Read the model definition and answer for the solid it produces. Units are mm, in the model's axes. A direction names the side the tool comes from. Give positions to 0.01 mm unless a question says otherwise; leave off trailing zeros. Loops run counter-clockwise (first coordinate to the right, second up) from the corner with the lowest first, then second, coordinate; pieces in that order, holes last. Notation, with made-up numbers: (84.5, -22) - (111.5, -22) arc R24 ccw to (111.5, 11) - close; hole circle Ø5 at (-3.75, -35). An arc over 180 degrees is marked (long way). Write item = value, one per line.
```python
from build123d import *

# Parameters (mm, degrees)
SKETCH1_W           = 27.4
SKETCH1_H           = 15.5
BOSS_EXTRUDE1_DEPTH = 9.6
FILLET1_R           = 2
SKETCH2_W           = 13
SKETCH2_H           = 4.45
BOSS_EXTRUDE2_DEPTH = 8
SKETCH3_W           = 0.5
SKETCH3_H           = 4.45
BOSS_EXTRUDE3_DEPTH = 35
CHAMFER1_SIZE       = 5
CHAMFER1_SIZE2      = 10.722534603


with BuildPart() as part:
    # Sketch1 → Boss-Extrude1 (new body)
    with BuildSketch(Plane(origin=(0, 0, 0), x_dir=(1, 0, 0), z_dir=(0, 1, 0))):
        with Locations((13.7, 7.75)):
            Rectangle(SKETCH1_W, SKETCH1_H)
    extrude(amount=BOSS_EXTRUDE1_DEPTH)

    # Fillet1
    fillet1_edges = [part.edges().sort_by_distance(p)[0] for p in [
        (0, 4.8, -15.5),
        (27.4, 4.8, -15.5),
        (27.4, 4.8, 0),
        (0, 4.8, 0),
    ]]
    fillet(fillet1_edges, radius=FILLET1_R)

    # Sketch2 → Boss-Extrude2 (add)
    with BuildSketch(Plane(origin=(0, 0, -15.5), x_dir=(-1, 0, 0), z_dir=(0, 0, -1))):
        with Locations((-10.5, 4.875)):
            Rectangle(SKETCH2_W, SKETCH2_H)
    extrude(amount=BOSS_EXTRUDE2_DEPTH)

    # Sketch3 → Boss-Extrude3 (add)
    with BuildSketch(Plane.ZY.offset(-4)):
        with Locations((-23.25, 4.875)):
            Rectangle(SKETCH3_W, SKETCH3_H)
    extrude(amount=BOSS_EXTRUDE3_DEPTH)

    # Chamfer1
    chamfer1_edges = [part.edges().sort_by_distance(p)[0] for p in [
        (17, 4.875, -23.5),
    ]]
    chamfer1_side = [part.faces().sort_by_distance(p)[0] for p in [
        (17, 4.875, -19.5),
    ]]
    chamfer(chamfer1_edges, length=CHAMFER1_SIZE, length2=CHAMFER1_SIZE2, reference=chamfer1_side[0])


solid = part.part
```
1) A cutting plane is placed at C-C on x = -5. Determine the outline of the cut face in (y, z), then the cut area to 4 significant figures.
Output:
outline = (2.65, -23.5) - (7.1, -23.5) - (7.1, -23) - (2.65, -23) - close
area = 2.225 mm²
2) The mould has two halves that part along Z. Classify faces 1 (the face through (4, 5, -19)), 2 (the face through (26.8, 4.87, -0.57)), 3 (the face through (6, 2.65, -20)): pulls with the +Z half, pulls with the -Z half, needs draft (parallel to the pull), parting line crosses it, or undercut.
Output:
face_1 = undercut
face_2 = pulls with the +Z half
face_3 = needs draft
3) Find the intervals of material crossed by probe 1 along X at (y, z) = (5.75, -10); probe 2 along Z at (x, y) = (7, 7.5); probe 3 along Z at (x, y) = (-17, 5.75), in increasing order.
Output:
probe_1 = 0 to 27.4
probe_2 = -15.5 to 0
probe_3 = -23.5 to -23
4) A cutting plane is placed at B-B on z = -17.25. Determine the outline of the cut face in (x, y).
Output:
outline = (4, 2.65) - (17, 2.65) - (17, 7.1) - (4, 7.1) - close
5) A tool of negligible diameter and unlimited length cuts with its end or side. For faces 4 (the face through (0, 5, -8)), 5 (the face through (6, 7.1, -20)), 6 (the face through (17, 5, -17)), from which of +Z, -Z, +X, -X, +Y, -Y can it reach the whole face along a straight path? Write none if from no direction.
Output:
face_4 = +Z, -X, +Y, -Y
face_5 = -Z, +X, -X, +Y
face_6 = -Z, +X, +Y, -Y
6) A cutting plane is placed at A-A on y = 2. Determine the outline of the cut face in (x, z).
Output:
outline = (0, -13.5) arc R2 ccw to (2, -15.5) - (25.4, -15.5) arc R2 ccw to (27.4, -13.5) - (27.4, -2) arc R2 ccw to (25.4, 0) - (2, 0) arc R2 ccw to (0, -2) - close
7) Each of these flat-tipped pins is pushed along its axis until it touches: P1, Ø2, axis at x = -6, y = 4, coming from the +Z side; P2, Ø1.3, axis at y = 4.5, z = -19.5, coming from the -X side; P3, Ø3.5, axis at y = 5, z = -17, coming from the +X side. Where does it stop, or does it pass through?
Output:
P1 = -23
P2 = 4
P3 = 26.37
8) A cutting plane is placed at D-D on y = 4.75. Determine the outline of the cut face in (x, z), then the cut area to 3 significant figures.
Output:
outline = (-31, -23.5) - (6.28, -23.5) - (17, -18.5) - (17, -15.5) - (25.4, -15.5) arc R2 ccw to (27.4, -13.5) - (27.4, -2) arc R2 ccw to (25.4, 0) - (2, 0) arc R2 ccw to (0, -2) - (0, -13.5) arc R2 ccw to (2, -15.5) - (4, -15.5) - (4, -23) - (-31, -23) - close
area = 516 mm²
